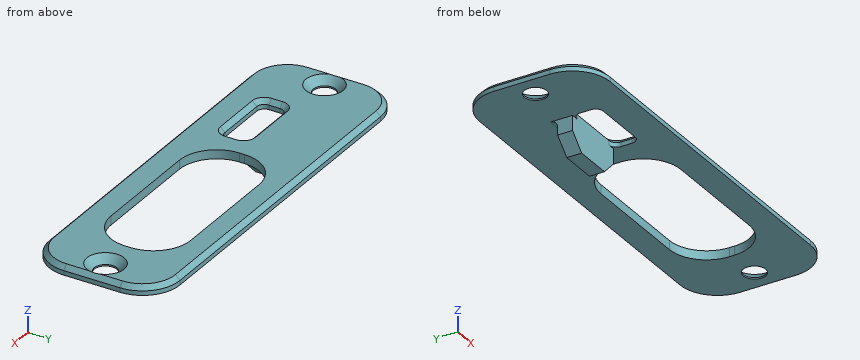
Autodesk Inventor part; units mm, degrees
ref_plane "YZ Plane" through (0, 0, 0) normal (1, 0, 0) x (0, 1, 0)
ref_plane "XZ Plane" through (0, 0, 0) normal (0, 1, 0) x (-1, 0, 0)
ref_plane "XY Plane" through (0, 0, 0) normal (0, 0, 1) x (1, 0, 0)
sketch "Sketch1" plane through (0, 0, 0) normal (0, 0, 1) x (1, 0, 0)
  line L0 (-27, 8.75) -> (27, 8.75)
  line L1 (27, 8.75) -> (27, -8.75)
  line L2 (27, -8.75) -> (-27, -8.75)
  line L3 (-27, -8.75) -> (-27, 8.75)
  point P0 (0, 0)
  dimension "d0" = 17.5
  dimension "d1" = 54
  dimension "d2" = 8.75
  dimension "d3" = 27
extrude "Extrusion1" add sketch "Sketch1" along normal blind 1.2
fillet "Fillet1" radius 5 4 edges at (-27, 8.75, 0.6) (-27, -8.75, 0.6) (27, 8.75, 0.6) (27, -8.75, 0.6)
sketch "Sketch2" plane through (0, 0, 1.2) normal (0, 0, 1) x (1, 0, 0)
  line L0 (-22, -8.75) -> (22, -8.75)
  line L1 (-27, 3.75) -> (-27, -3.75)
  line L2 (27, -3.75) -> (27, 3.75)
  point P0 (0, 0)
  point P1 (-24, 0)
  point P2 (24, 0)
  dimension "d7" = 8.75
  dimension "d8" = 8.75
  dimension "d9" = 3
  dimension "d10" = 3
hole "Hole1" at (-24, 0, 1.2) at (24, 0, 1.2) direction (0, 0, -1) diameter 3 depth 8.8 tip angle 118 countersink diameter 5 countersink angle 90
chamfer "Chamfer1" distance 0.6 angle 45 8 edges at (0, 8.75, 1.2) (-25.5355, 7.2855, 1.2) (-27, 0, 1.2) (-25.5355, -7.2855, 1.2) (0, -8.75, 1.2) (25.5355, -7.2855, 1.2) (27, 0, 1.2) (25.5355, 7.2855, 1.2)
sketch "Sketch3" plane through (0, 0, 1.2) normal (0, 0, 1) x (1, 0, 0)
  line L0 (-21, 6.75) -> (21, 6.75)
  line L1 (21, 6.75) -> (21, -6.75)
  line L2 (21, -6.75) -> (-21, -6.75)
  line L3 (-21, -6.75) -> (-21, 6.75)
  line L4 (22, 8.75) -> (-22, 8.75)
  line L5 (-22, -8.75) -> (22, -8.75)
  line L6 (-27, 3.75) -> (-27, -3.75)
  line L7 (27, -3.75) -> (27, 3.75)
  line L8 (-17.6, -1.05) -> (-8.6, -1.05)
  line L9 (-8.6, -1.05) -> (-8.6, -4.55)
  line L10 (-8.6, -4.55) -> (-17.6, -4.55)
  line L11 (-17.6, -4.55) -> (-17.6, -1.05)
  point P0 (0, 0)
  dimension "d21" = 2
  dimension "d22" = 2
  dimension "d23" = 6
  dimension "d24" = 6
  dimension "d25" = 3.4
  dimension "d26" = 9
  dimension "d27" = 3.5
  dimension "d28" = 2.2
extrude "Extrusion2" cut sketch "Sketch3" against normal blind 1.2 contours L8 L9 L10 L11
sketch "Sketch4" plane through (0, 0, 1.2) normal (0, 0, 1) x (1, 0, 0)
  line L0 (-5.6, 5.55) -> (19.4, 5.55)
  line L1 (19.4, 5.55) -> (19.4, -5.15)
  line L2 (19.4, -5.15) -> (-5.6, -5.15)
  line L3 (-5.6, -5.15) -> (-5.6, 5.55)
  line L4 (22, 8.75) -> (-22, 8.75)
  line L5 (-27, 3.75) -> (-27, -3.75)
  line L6 (-8.6, -4.55) -> (-17.6, -4.55)
  point P0 (0, 0)
  dimension "d31" = 25
  dimension "d32" = 10.7
  dimension "d34" = 21.4
  dimension "d35" = 3.2
  dimension "d36" = 0.6
extrude "Extrusion3" cut sketch "Sketch4" against normal blind 1.2
fillet "Fillet2" radius 5 4 edges at (-5.6, 5.55, 0.6) (-5.6, -5.15, 0.6) (19.4, 5.55, 0.6) (19.4, -5.15, 0.6)
fillet "Fillet3" radius 1 4 edges at (-8.6, -1.05, 0.6) (-17.6, -1.05, 0.6) (-17.6, -4.55, 0.6) (-8.6, -4.55, 0.6)
sketch "Sketch5" plane through (0, 0, 0) normal (0, 0, -1) x (-1, 0, 0)
  line L0 (8.6, 0.95) -> (17.6, 0.95)
  line L1 (17.6, 0.95) -> (17.6, -1.05)
  line L2 (17.6, -1.05) -> (8.6, -1.05)
  line L3 (8.6, -1.05) -> (8.6, 0.95)
  line L4 (9.6, -1.05) -> (16.6, -1.05)
  line L5 (8.6, -3.55) -> (8.6, -2.05)
  line L6 (17.6, -2.05) -> (17.6, -3.55)
  point P0 (0, 0)
  dimension "d47" = 2
extrude "Extrusion4" add sketch "Sketch5" along normal blind 4
fillet "Fillet4" radius 1 1 edges at (-13.1, 0.95, 0)
chamfer "Chamfer4" distance 2 angle 45 2 edges at (-8.6, -0.05, -4) (-17.6, -0.05, -4)
chamfer "Chamfer6" distance 0.6 angle 45 8 edges at (-13.1, -1.05, 1.2) (-8.8929, -1.3429, 1.2) (-8.6, -2.8, 1.2) (-8.8929, -4.2571, 1.2) (-13.1, -4.55, 1.2) (-17.3071, -4.2571, 1.2) (-17.6, -2.8, 1.2) (-17.3071, -1.3429, 1.2)
properties part number "cover"
Input: part model. Units: mm. Frame: model coordinates. Round coordinates to 2 decimals unless told otherwise and drop trailing zeros. Loops run counter-clockwise (first coordinate to the right, second up) from the corner with the lowest first, then second, coordinate; pieces in that order, holes last. Notation, with made-up numbers: (34, 51.5) - (72, 51.5) arc R29 ccw to (72, 75.5) - close; hole circle Ø8 at (35.5, 54.25). An arc over 180 degrees is marked (long way). One line per item, written item: value. Start each with the question number.
(1) Section B-B, the plane z = -2.95. Return loops of the section in (x, y).
(2) Contact query for flat-ended pins moving along their axis: P1, Ø2.5, axis at x = -24, y = 0, coming from the -Z side; P2, Ø4, axis at x = 19, y = 2, coming from the +Z side; P3, Ø5, axis at x = 24, y = 0, coming from the -Z side; P4, Ø1.6, axis at y = 1, z = -1, coming from the -X side. Output: stop coordinate, or through.
(3) Section A-A, the plane x = 5. Return loops of the section in (y, z), plus the area to 3 significant figures.
(4) Ray query, line 1 (X direction, y = 0, z = 0.15); line 2 (Y direction, x = -15, z = -3.05); line 3 (Y direction, x = 14.5, z = 0.15). Return the intervals inside material, ascending. Write a range as [from, to].
Results below:
1. outline: (-16.65, -1.05) - (-9.55, -1.05) - (-9.55, 0.95) - (-16.65, 0.95) - close
2. P1: through
2. P2: z = 1.2
2. P3: z = 0
2. P4: x = -17.6
3. outline: (-8.75, 0) - (-5.15, 0) - (-5.15, 1.2) - (-8.15, 1.2) - (-8.75, 0.6) - close; (5.55, 0) - (8.75, 0) - (8.75, 0.6) - (8.15, 1.2) - (5.55, 1.2) - close
3. area: 7.80 mm^2
4. line 1: [-27, -25.5], [-22.5, -5.6], [19.4, 22.5], [25.5, 27]
4. line 2: [-1.05, 0.95]
4. line 3: [-8.75, -5.15], [5.55, 8.75]
